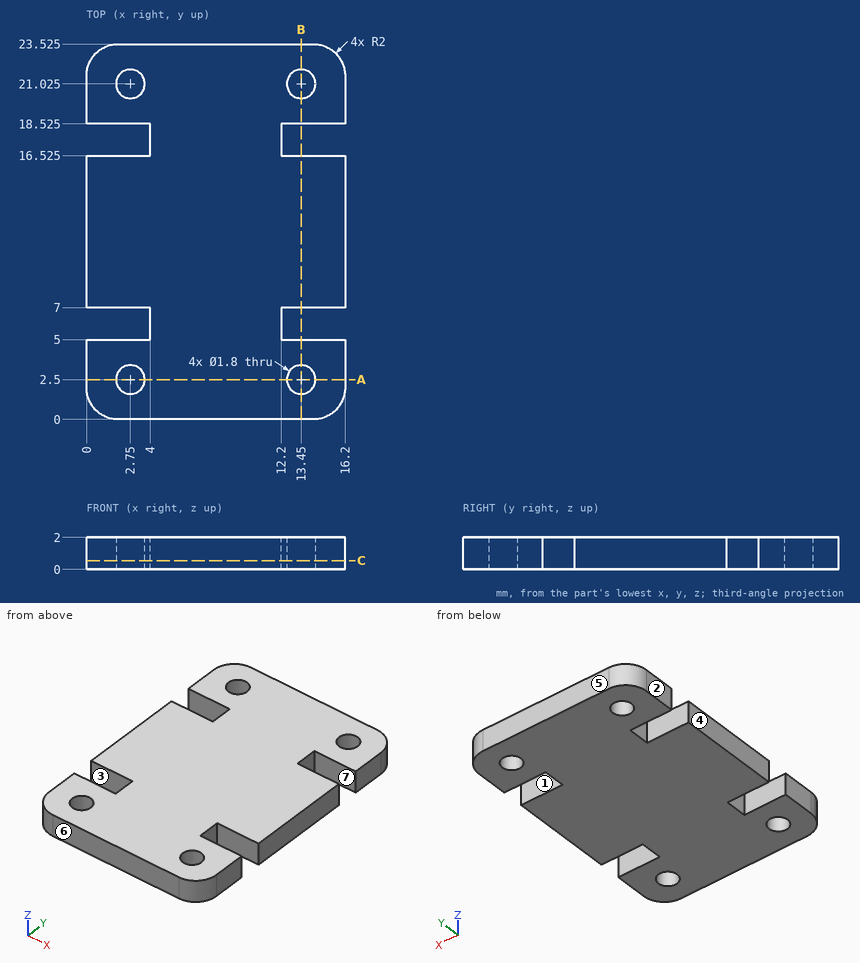
Verification items for this drawing (mm, ordinates from the low corner). A direction names the side the tool comes from. Coordinates: 2 decimals unless noted, no trailing zeros. Order: outer loops, then holes, each group sorted by start corner. A loop starts at its lowest first (then second) coordinate and runs counter-clockwise, first axis right, second up. Notation, with made-up numbers: M -40,-39 L 18,-39 A22 ccw 18,-26 Z; hole C 11,79.5 d5. An arc over 180 degrees is marked long. One line per item, written item: value. Start each with the question number.
Item 1: Depth check by flat-ended pin: P1, Ø0.6, axis at y = 5.5, z = 1, coming from the +X side. Enter the tip coordinate at first touch or a pass-through.
Item 2: Sectioned sample at A-A on y = 2.5. Record the cut outline in (x, z), then the cut area to 3 significant figures.
Item 3: Sectioned sample at B-B on x = 13.45. Record the cut outline in (y, z) (3 decimals), then the cut area to 4 significant figures.
Item 4: Thickness scan on probe 1 along Y at (x, z) = (12.5, 1.1) (3 decimals); probe 2 along Y at (x, z) = (13.45, 1.5) (3 decimals); probe 3 along Y at (x, z) = (14.75, 0.2) (3 decimals). Record the ranges inside material, lowest first.
Item 5: Access from +Z, -Z, +X, -X, +Y, -Y to the whole of each face (thin tool, end or side, straight path). Record for the marked faces 1, 2 and 3.
Item 6: Sectioned sample at C-C on z = 0.55. Record the cut outline in (x, y) (3 decimals).
Item 7: Mould release check, pull along Y, two halves, no side actions. Record for the marked faces 4, 5, 6 and 7: pulls with the +Y half, pulls with the -Y half, needs draft (parallel to the pull), parting line crosses it, or undercut.
Calculated:
1. P1: x = 12.2
2. outline: M 0,0 L 1.85,0 L 1.85,2 L 0,2 Z; M 3.65,0 L 12.55,0 L 12.55,2 L 3.65,2 Z; M 14.35,0 L 16.2,0 L 16.2,2 L 14.35,2 Z
2. area: 25.2 mm^2
3. outline: M 0,0 L 1.6,0 L 1.6,2 L 0,2 Z; M 3.4,0 L 5,0 L 5,2 L 3.4,2 Z; M 7,0 L 16.525,0 L 16.525,2 L 7,2 Z; M 18.525,0 L 20.125,0 L 20.125,2 L 18.525,2 Z; M 21.925,0 L 23.525,0 L 23.525,2 L 21.925,2 Z
3. area: 31.85 mm^2
4. probe 1: 0 to 5, 7 to 16.525, 18.525 to 23.525
4. probe 2: 0 to 1.6, 3.4 to 5, 7 to 16.525, 18.525 to 20.125, 21.925 to 23.525
4. probe 3: 0.077 to 5, 7 to 16.525, 18.525 to 23.448
5. face 1: +Z, -Z, +X
5. face 2: +Z, -Z, -X, +Y, -Y
5. face 3: +Z, -Z, -X
6. outline: M 0,2 A2 ccw 2,0 L 14.2,0 A2 ccw 16.2,2 L 16.2,5 L 12.2,5 L 12.2,7 L 16.2,7 L 16.2,16.525 L 12.2,16.525 L 12.2,18.525 L 16.2,18.525 L 16.2,21.525 A2 ccw 14.2,23.525 L 2,23.525 A2 ccw 0,21.525 L 0,18.525 L 4,18.525 L 4,16.525 L 0,16.525 L 0,7 L 4,7 L 4,5 L 0,5 Z; hole C 2.75,2.5 d1.8; hole C 2.75,21.025 d1.8; hole C 13.45,2.5 d1.8; hole C 13.45,21.025 d1.8
7. face 4: needs draft
7. face 5: pulls with the +Y half
7. face 6: pulls with the -Y half
7. face 7: undercut
